Autodesk Inventor part; units mm, degrees
ref_plane "YZ Plane" through (0, 0, 0) normal (1, 0, 0) x (0, 1, 0)
ref_plane "XZ Plane" through (0, 0, 0) normal (0, 1, 0) x (-1, 0, 0)
ref_plane "XY Plane" through (0, 0, 0) normal (0, 0, 1) x (1, 0, 0)
sketch "Esquisse1" plane through (0, 0, 0) normal (0, 1, 0) x (-1, 0, 0)
  line L0 (0, -42) -> (0, 42) construction
  circle A0 centre (0, 0) radius 30
  circle A1 centre (22, 0) radius 2.5
  circle A2 centre (11, 19.0526) radius 2.5
  circle A3 centre (-11, 19.0526) radius 2.5
  circle A4 centre (-22, 0) radius 2.5
  circle A5 centre (-11, -19.0526) radius 2.5
  circle A6 centre (11, -19.0526) radius 2.5
  line L1 (17.9263, -5.3263) -> (22, 0) construction
  line L2 (-2.5, -16.1785) -> (-12.761, -10.2543)
  line L3 (-15.261, -5.9242) -> (-15.261, 5.9242)
  line L4 (-12.761, 10.2543) -> (-2.5, 16.1785)
  line L5 (2.5, 16.1785) -> (12.761, 10.2543)
  line L6 (15.261, 5.9242) -> (15.261, -5.9242)
  line L7 (12.761, -10.2543) -> (2.5, -16.1785)
  arc A7 (2.5, 16.1785) -> (-2.5, 16.1785) centre (0, 11.8484) ccw
  arc A8 (15.261, 5.9242) -> (12.761, 10.2543) centre (10.261, 5.9242) ccw
  arc A9 (12.761, -10.2543) -> (15.261, -5.9242) centre (10.261, -5.9242) ccw
  arc A10 (-2.5, -16.1785) -> (2.5, -16.1785) centre (0, -11.8484) ccw
  arc A11 (-15.261, -5.9242) -> (-12.761, -10.2543) centre (-10.261, -5.9242) ccw
  arc A12 (-12.761, 10.2543) -> (-15.261, 5.9242) centre (-10.261, 5.9242) ccw
  line L8 (0, 0) -> (10.261, -5.9242) construction
  line L9 (22, 0) -> (0, 0) construction
  point P0 (0, -17.6219)
  point P1 (-15.261, -8.8109)
  point P2 (-15.261, 8.8109)
  point P3 (0, 17.6219)
  point P4 (15.261, 8.8109)
  point P5 (15.261, -8.8109)
  dimension "d0" = 60
  dimension "d6" = 360
  dimension "d10" = 22
  dimension "d21" = 5
  dimension "d30" = 5
  dimension "d31" = 30
extrude "Extrusion1" add sketch "Esquisse1" against normal blind 3.175
equation "\"d8\" = d_aluminum_thickness"
equation "\"d_profile_section\" = 40"
equation "\"d_prfc_thickness\" = 3"
equation "\"d_front_arm_od\" = 31.75"
equation "\"d_front_arm_id\" = 29.2608"
equation "\"d_arm_length\" = 250"
equation "\"d_suspension_height\" = 140"
equation "\"d_aluminum_thickness\" = 3.175"
equation "\"d_suspension_box_width\" = 40"
equation "\"d_wheelbase\" = 1600"
equation "\"a_tilt\" = 10deg"
equation "\"d_rear_profile_width\" = 50.8"
equation "\"d_rear_profile_height\" = 101.6"
equation "\"d_central_profile_width\" = 50.8"
equation "\"d_central_profile_height\" = 101.6"
equation "\"d_handle_bar_od\" = 38.1"
equation "\"d_handle_bar_id\" = 30"
equation "\"a_direction_column\" = 35deg"
equation "\"front_suspension_height\" = 140.92977"
equation "\"front_suspension_width\" = 150"
equation "\"a_caster_angle\" = 25deg"
equation "\"d_handlebar_arm_length\" = 80"
equation "\"d_handlebar_pivot_offset\" = 65"
equation "\"a_handlebar_angle\" = 60deg"
equation "\"d_left_to_right_front_pivots\" = 28"
equation "\"d_aluminum_bar_thickness\" = 12.7"
equation "\"d_steering_arm_length\" = 70"
equation "\"d_steering_height_from_hub_carrier_center\" = 18"
equation "\"d_central_beam_inclination\" = 12"
equation "\"a_central_beam_inclination\" = 12deg"
equation "\"d_central_beam_screws_diameter\" = 8"
equation "\"d_rear_profile_wall_thickness\" = 4.7625"
equation "\"d_rear_profile_wall_thickness_1\" = 4.7625"
equation "\"d_central_pivot_screw_diameter\" = 15.875"
properties part number "Wheel_external_hub_ring" material "Aluminium 6061"
Geometry check sheet. Reference: the model listing, model coordinates, mm. A direction names the side the tool comes from. Give positions to 0.01 mm unless a question says otherwise; leave off trailing zeros. Loops run counter-clockwise (first coordinate to the right, second up) from the corner with the lowest first, then second, coordinate; pieces in that order, holes last. Notation, with made-up numbers: M 43,49 L 47,49 A18 cw 47,80 Z; hole C 55,-19.75 d6. An arc over 180 degrees is marked long. Answer as a JSON object with one key per item and string values. Group by question number.
Item 1: Sectioned sample at C-C on x = 11. Record the boundary of the cut face in (y, z) (3 decimals).
Item 2: Sectioned sample at B-B on z = -20. Record the boundary of the cut face in (x, y) (3 decimals).
Item 3: Sectioned sample at A-A on z = 0. Record the boundary of the cut face in (x, y) (3 decimals), plus the area to 3 significant figures.
Item 4: Gauge pin test, flat ends, axial feed: pin 1 (12 mm diameter, centred on x = -22.5, z = -19, fed in from +Y); pin 2 (1.6 mm diameter, centred on y = -2, z = 1.5, fed in from +X); pin 3 (1 mm diameter, centred on y = -1.5, z = -22, fed in from -X); pin 4 (1 mm diameter, centred on y = -1.5, z = -16.5, fed in from +X). Record the tip position at first contact, or that the pin passes through.
Item 5: Sectioned sample at D-D on y = -1.25. Record the boundary of the cut face in (x, z).
Item 6: Material ranges on L1, parallel to X at y = -2.9, z = -17.5; L2, parallel to X at y = -2.55, z = 0.5; L3, parallel to Z at x = -11, y = -2.4, recorded low to high.
Item 7: Mould release check, pull along Z, two halves, no side actions. Record for faces 3 (the flat face through (7, 0, 14)), 4 (the cylindrical face through (11.33, -1.57, 21.53)), 5 (the cylindrical face through (29.97, -1.57, 1.32)): pulls with the +Z half, pulls with the -Z half, needs draft (parallel to the pull), parting line crosses it, or undercut.
Item 8: Access from +Z, -Z, +X, -X, +Y, -Y to the whole of each face (thin tool, end or side, straight path). Record for faces 1 (the flat face through (7, -3.175, 14)), 2 (the flat face through (7.559, -1.565, -13.258)).
Findings below:
{
 "1": {"outline": "M -3.175,-27.911 L 0,-27.911 L 0,-21.553 L -3.175,-21.553 Z; M -3.175,-16.553 L 0,-16.553 L 0,-11.271 L -3.175,-11.271 Z; M -3.175,11.271 L 0,11.271 L 0,16.553 L -3.175,16.553 Z; M -3.175,21.553 L 0,21.553 L 0,27.911 L -3.175,27.911 Z"},
 "2": {"outline": "M -22.361,-3.175 L -13.314,-3.175 L -13.314,0 L -22.361,0 Z; M -8.686,-3.175 L 8.686,-3.175 L 8.686,0 L -8.686,0 Z; M 13.314,-3.175 L 22.361,-3.175 L 22.361,0 L 13.314,0 Z"},
 "3": {"outline": "M -30,-3.175 L -24.5,-3.175 L -24.5,0 L -30,0 Z; M -19.5,-3.175 L -15.261,-3.175 L -15.261,0 L -19.5,0 Z; M 15.261,-3.175 L 19.5,-3.175 L 19.5,0 L 15.261,0 Z; M 24.5,-3.175 L 30,-3.175 L 30,0 L 24.5,0 Z", "area": "61.8 mm2"},
 "4": {"pin 1": "y = 0", "pin 2": "x = 29.99", "pin 3": "x = -20.92", "pin 4": "x = 25.38"},
 "5": {"outline": "C 0,0 d60; hole C -22,0 d5; hole M -15.26,-5.92 A5 ccw -12.76,-10.25 L -2.5,-16.18 A5 ccw 2.5,-16.18 L 12.76,-10.25 A5 ccw 15.26,-5.92 L 15.26,5.92 A5 ccw 12.76,10.25 L 2.5,16.18 A5 ccw -2.5,16.18 L -12.76,10.25 A5 ccw -15.26,5.92 Z; hole C -11,-19.05 d5; hole C -11,19.05 d5; hole C 11,-19.05 d5; hole C 11,19.05 d5; hole C 22,0 d5"},
 "6": {"L1": "-24.37 to -12.96, -9.04 to 9.04, 12.96 to 24.37", "L2": "-30 to -24.45, -19.55 to -15.26, 15.26 to 19.55, 24.45 to 30", "L3": "-27.91 to -21.55, -16.55 to -11.27, 11.27 to 16.55, 21.55 to 27.91"},
 "7": {"face 3": "needs draft", "face 4": "undercut", "face 5": "parting line crosses it"},
 "8": {"face 1": "+Z, -Z, +X, -X, -Y", "face 2": "+Y, -Y"}
}
